Model file for the job. Use its own axes, mm. Round coordinates to 2 decimals unless told otherwise and drop trailing zeros. Loops run counter-clockwise (first coordinate to the right, second up) from the corner with the lowest first, then second, coordinate; pieces in that order, holes last. Notation, with made-up numbers: M 17.25,20.5 L 29.25,20.5 A15 cw 29.25,31.5 Z; hole C 24.5,53.25 d2. An arc over 180 degrees is marked long. Use a Markdown table: item, result. Add a question column.
Item 1: Saw through at C-C on y = 0. Write the cut outline in (x, z).
Item 2: Saw through at D-D on x = 91. Write the cut outline in (y, z), then the cut area to 3 significant figures.
Item 3: Saw through at A-A on y = 16. Write the cut outline in (x, z).
Item 4: Pin check, flat tips, straight feed: P1, Ø1.5, axis at y = 17.5, z = 3, coming from the +X side; P2, Ø3, axis at x = 75, y = 0, coming from the +Z side; P3, Ø2, axis at x = 24, z = 2, coming from the +Y side. Stop position of each tip, or through.
Item 5: Saw through at B-B on z = 3.25. Write the cut outline in (x, y).
Item 6: Wall check: L1, parallel to Y at x = -45, z = 1; L2, parallel to Y at x = -29, z = 2.15; L3, parallel to X at y = 18, z = 2.85. Give the ranges that are in metal, low to high. Write a range as from..to.
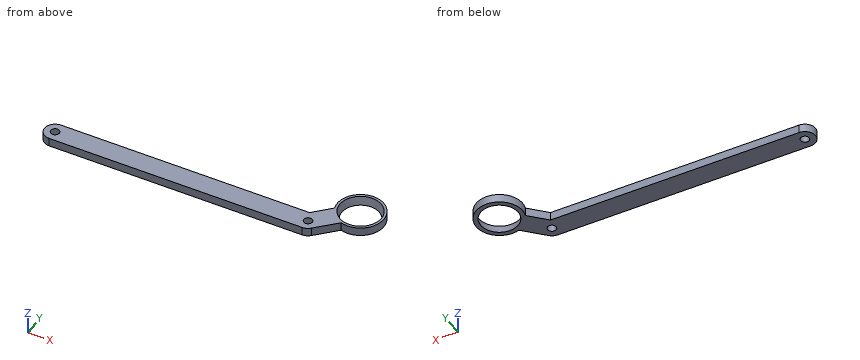
```python
from build123d import *

# Parameters (mm, degrees)
SKETCH1_R           = 2
SKETCH1_R_2         = 8.8
BOSS_EXTRUDE1_DEPTH = 4
SKETCH2_R           = 9.8
CUT_EXTRUDE2_DEPTH  = 4
CUT_EXTRUDE2_DRAFT  = -13


with BuildPart() as part:
    # Sketch1 → Boss-Extrude1 (new body)
    with BuildSketch(Plane.XY):
        with BuildLine():
            ThreePointArc((75, -5), (76.913417162, -4.619397663), (78.535533906, -3.535533906))
            Line((78.535533906, -3.535533906), (87.607330676, 5.536262864))
            ThreePointArc((87.607330676, 5.536262864), (98.778174593, 23.778174593), (80.536262864, 12.607330676))
            Line((80.536262864, 12.607330676), (72.928932188, 5))
            Line((72.928932188, 5), (-45, 5))
            ThreePointArc((-45, 5), (-50, 0), (-45, -5))
            Line((-45, -5), (75, -5))
        make_face()
        with Locations((-45, 0)):
            Circle(SKETCH1_R, mode=Mode.SUBTRACT)
        with Locations((75, 0)):
            Circle(SKETCH1_R, mode=Mode.SUBTRACT)
        with Locations((91, 16)):
            Circle(SKETCH1_R_2, mode=Mode.SUBTRACT)
    extrude(amount=BOSS_EXTRUDE1_DEPTH)


with BuildPart() as cut_extrude2_tool:
    # Sketch2 → Cut-Extrude2 (with draft: the straight prism first)
    with BuildSketch(Plane.XY.offset(4)):
        with Locations((91, 16)):
            Circle(SKETCH2_R)
    extrude(amount=-CUT_EXTRUDE2_DEPTH)
    # Cut-Extrude2: the draft: its side faces are tilted about the plane it starts from
    cut_extrude2_sides = [cut_extrude2_tool.faces().sort_by_distance(p)[0] for p in [
        (81.2, 16, 2),
    ]]
    draft(cut_extrude2_sides, Plane.XY.offset(4), CUT_EXTRUDE2_DRAFT)


with BuildPart() as part_1:
    add(part.part)

    # Cut-Extrude2: cut by cut_extrude2_tool
    add(cut_extrude2_tool.part, mode=Mode.SUBTRACT)


solid = part_1.part
```
Entries:
| question | item | result |
|---|---|---|
| 1 | outline | M -50,0 L -47,0 L -47,4 L -50,4 Z; M -43,0 L 73,0 L 73,4 L -43,4 Z; M 77,0 L 82.07,0 L 82.07,4 L 77,4 Z |
| 2 | outline | M 5,0 L 7.12,0 L 6.2,4 L 5,4 Z; M 24.88,0 L 27,0 L 27,4 L 25.8,4 Z |
| 2 | area | 13.3 mm2 |
| 3 | outline | M 80,0 L 82.12,0 L 81.2,4 L 80,4 Z; M 99.88,0 L 102,0 L 102,4 L 100.8,4 Z |
| 4 | P1 | x = 101.97 |
| 4 | P2 | through |
| 4 | P3 | y = 5 |
| 5 | outline | M -45,-5 L 75,-5 A5 ccw 78.54,-3.54 L 87.61,5.54 A11 ccw long 80.54,12.61 L 72.93,5 L -45,5 A5 ccw Z; hole C -45,0 d4; hole C 75,0 d4; hole C 91,16 d19.25 |
| 6 | L1 | -5..-2, 2..5 |
| 6 | L2 | -5..5 |
| 6 | L3 | 80.18..81.68, 100.32..101.82 |
